Source: CAD feature listing. Evaluate the final solid. Frame: model axes, mm. Face numbers are marked on the shaded views. A direction names the side the tool comes from. Round coordinates to 2 decimals unless told otherwise and drop trailing zeros. Write each loop counter-clockwise with the first axis right and the second up, starting at its lowest first coordinate (ties: lowest second). Pieces come first, ordered by that corner, then holes.
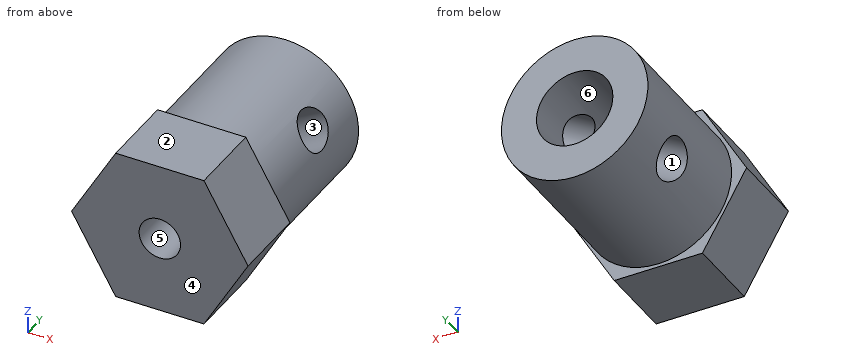
```python
from build123d import *

# Parameters (mm, degrees)
EXTRUDE_1_DEPTH     = 6
SKETCH_2_R          = 5.75
EXTRUDE_2_DEPTH     = 12
SKETCH_3_R          = 1.625
CUT_EXTRUDE_1_DEPTH = 300
SKETCH_4_R          = 3
CUT_EXTRUDE_2_DEPTH = 12
SKETCH_5_R          = 1.625
CUT_EXTRUDE_3_DEPTH = 12


with BuildPart() as part:
    # Эскиз1 → Бобышка-Вытянуть1 (new body)
    with BuildSketch(Plane(origin=(0, 0, 0), x_dir=(1, 0, 0), z_dir=(0, 1, 0))):
        Polygon((6.92820323, 0), (3.464101615, 6), (-3.464101615, 6), (-6.92820323, 0), (-3.464101615, -6), (3.464101615, -6), align=None)
    extrude(amount=EXTRUDE_1_DEPTH)

    # Эскиз2 → Бобышка-Вытянуть2 (add)
    with BuildSketch(Plane(origin=(0, 6, 0), x_dir=(1, 0, 0), z_dir=(0, 1, 0))):
        with Locations(Location((0, 0, 0), (0, 0, 270))):
            Circle(SKETCH_2_R)
    extrude(amount=EXTRUDE_2_DEPTH)

    # Эскиз3 → Вырез-Вытянуть1 (cut)
    with BuildSketch(Plane.XZ):
        with Locations(Location((0, 0, 0), (0, 0, 270))):
            Circle(SKETCH_3_R)
    extrude(amount=-CUT_EXTRUDE_1_DEPTH, mode=Mode.SUBTRACT)

    # Эскиз4 → Вырез-Вытянуть2 (cut)
    with BuildSketch(Plane(origin=(0, 18, 0), x_dir=(1, 0, 0), z_dir=(0, 1, 0))):
        with Locations(Location((0, 0, 0), (0, 0, 270))):
            Circle(SKETCH_4_R)
    extrude(amount=-CUT_EXTRUDE_2_DEPTH, mode=Mode.SUBTRACT)

    # Эскиз5 → Вырез-Вытянуть3 (cut)
    with BuildSketch(Plane(origin=(-5.196152423, 0, -3), x_dir=(-0.5000000000000003, 0, 0.8660254037844386), z_dir=(-0.8660254037844385, 0, -0.5000000000000002))):
        with Locations((0, 13)):
            Circle(SKETCH_5_R)
    extrude(amount=-CUT_EXTRUDE_3_DEPTH, mode=Mode.SUBTRACT)


solid = part.part
```
Q1. Line query: line 1 (X direction, y = 11.5, z = 0); line 2 (Z direction, x = -2.5, y = 15.75); line 3 (Z direction, x = -2, y = 8.75). Output: solid intervals per line, ascending.
Q2. Section query B-B, the plane y = 13.75. Output: boundary loops of the cut face in (x, z).
Q3. Section query C-C, the plane y = 16.25. Output: boundary loops of the cut face in (x, z).
Q4. Pin query (flat end, axial travel): P1, Ø1.5, axis at y = 8.5, z = 4.5, coming from the -X side; P2, Ø4, axis at y = 5.5, z = -1.5, coming from the -X side; P3, Ø5, axis at x = -2.5, y = 16, coming from the +Z side; P4, Ø3, axis at x = 3.5, y = 10, coming from the -Z side. Return the tip coordinate at first contact, or that it passes through.
Q5. Set-up query: the marked faces 5 and 6. Return all of +Z, -Z, +X, -X, +Y, -Y with unobstructed straight access to the full face (end or side cutting, diameter ignored); none if empty.
Q6. Section query A-A, the plane x = 0. Output: boundary loops of the cut face in (y, z) (3 decimals), and give its area (4 significant figures).
Q7. Mould query, pull axis Y, two halves, no side actions, for the marked faces 1, 2, 3 and 4. Classes: pulls with the +Y half, pulls with the -Y half, needs draft (parallel to the pull), parting line crosses it, or undercut.
Filled in:
1. line 1: x = -5.75 to -3, 3 to 5.75
1. line 2: z = -5.18 to -1.66, 1.66 to 5.18
1. line 3: z = -5.39 to -2.24, 2.24 to 5.39
2. outline: (-5.54, -1.53) - (-3, -0.07) arc R3 cw to (1.56, 2.56) - (4.1, 4.03) arc R5.75 ccw to start; (-4.1, -4.03) arc R5.75 ccw to (5.54, 1.53) - (3, 0.07) arc R3 cw to (-1.56, -2.56) - close
3. outline: circle Ø11.5 at (0, 0); hole circle Ø6 at (0, 0)
4. P1: stops at x = -4.36
4. P2: stops at x = -6.93
4. P3: stops at z = 5.75
4. P4: stops at z = -5.39
5. face 5: +Y, -Y
5. face 6: +Y
6. outline: (0, -6) - (6, -6) - (6, -5.75) - (18, -5.75) - (18, -3) - (6, -3) - (6, -1.625) - (0, -1.625) - close; (0, 1.625) - (6, 1.625) - (6, 3) - (18, 3) - (18, 5.75) - (6, 5.75) - (6, 6) - (0, 6) - close
6. area: 118.5 mm2
7. face 1: undercut
7. face 2: needs draft
7. face 3: undercut
7. face 4: pulls with the -Y half
